Source: three-view drawing plus pictorial views. Frame: mm from the lowest corner of the part. A direction names the side the tool comes from. Coordinates: 2 decimals unless noted, no trailing zeros. Loops run counter-clockwise (first coordinate to the right, second up) from the corner with the lowest first, then second, coordinate; pieces in that order, holes last. Notation, with made-up numbers: (-29, 48.25) - (-4, 48.25) arc R21 cw to (-4, 55.25) - close; hole circle Ø7 at (-32.75, 49). An arc over 180 degrees is marked (long way). Return JSON: item names as keys, results as strings.
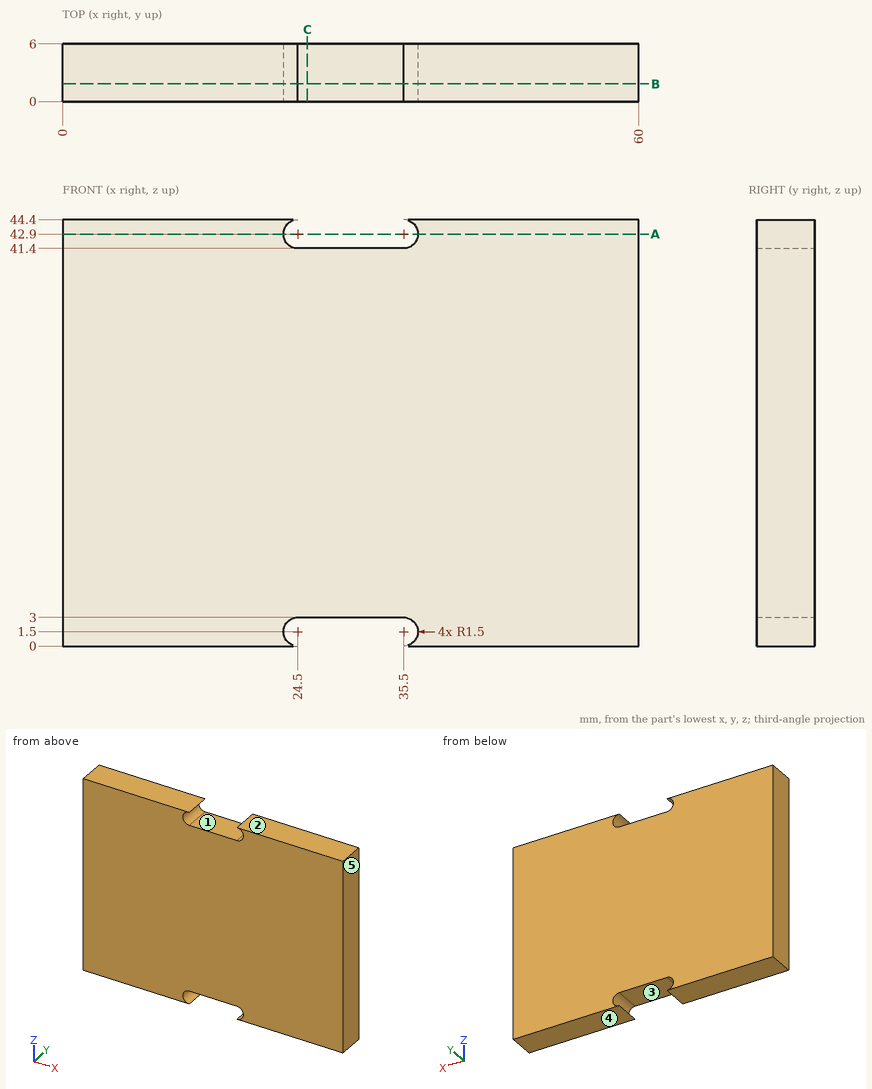
Item 1: Mould query, pull axis X, two halves, no side actions, for the marked faces 3, 4 and 5. Classes: +X half, -X half, draft (parallel to the pull), parting line (faces both ways), or undercut.
Worked out:
{"face 3": "undercut", "face 4": "draft", "face 5": "+X half"}
Item 2: Section query C-C, the plane x = 25.5. Return loops of the section in (y, z), and give its area (3 significant figures).
Worked out:
{"outline": "(0, 3) - (6, 3) - (6, 41.4) - (0, 41.4) - close", "area": "230 mm^2"}
Item 3: Section query B-B, the plane y = 1.85. Return loops of the section in (x, z), and give its area (3 significant figures).
Worked out:
{"outline": "(0, 0) - (24.5, 0) arc R1.5 cw to (24.5, 3) - (35.5, 3) arc R1.5 cw to (35.5, 0) - (60, 0) - (60, 44.4) - (35.5, 44.4) arc R1.5 cw to (35.5, 41.4) - (24.5, 41.4) arc R1.5 cw to (24.5, 44.4) - (0, 44.4) - close", "area": "2,580 mm^2"}
Item 4: Reachability of the marked faces 1 and 2 from +Z, -Z, +X, -X, +Y, -Y: full face, straight path, thin tool, end or side. Return the list, or none.
Worked out:
{"face 1": "+Z, +Y, -Y", "face 2": "+Z, +X, -X, +Y, -Y"}
Item 5: Ray query, probe 1 along Z at (x, y) = (31.5, 0.5). Return the intervals inside material, ascending. Write a range as from..to.
Worked out:
{"probe 1": "3..41.4"}
Item 6: First-contact query: pin 1 Ø1.8 at (x, y) = (32.5, 2) entering from +Z; pin 2 Ø3 at (x, y) = (28, 3) entering from -Z. Flat tips, straight axial feed; report the tip coordinate or a pass-through.
Worked out:
{"pin 1": "z = 41.4", "pin 2": "z = 3"}
Item 7: Section query A-A, the plane z = 42.9. Return loops of the section in (x, y).
Worked out:
{"outline": "(0, 0) - (23, 0) - (23, 6) - (0, 6) - close; (37, 0) - (60, 0) - (60, 6) - (37, 6) - close"}
